Could you check a few things on this drawing? It's one solid part, dimensions in mm from its lowest x, y, z. Give positions to 0.01 mm unless a question says otherwise; leave off trailing zeros. Use a Markdown table: item, result.
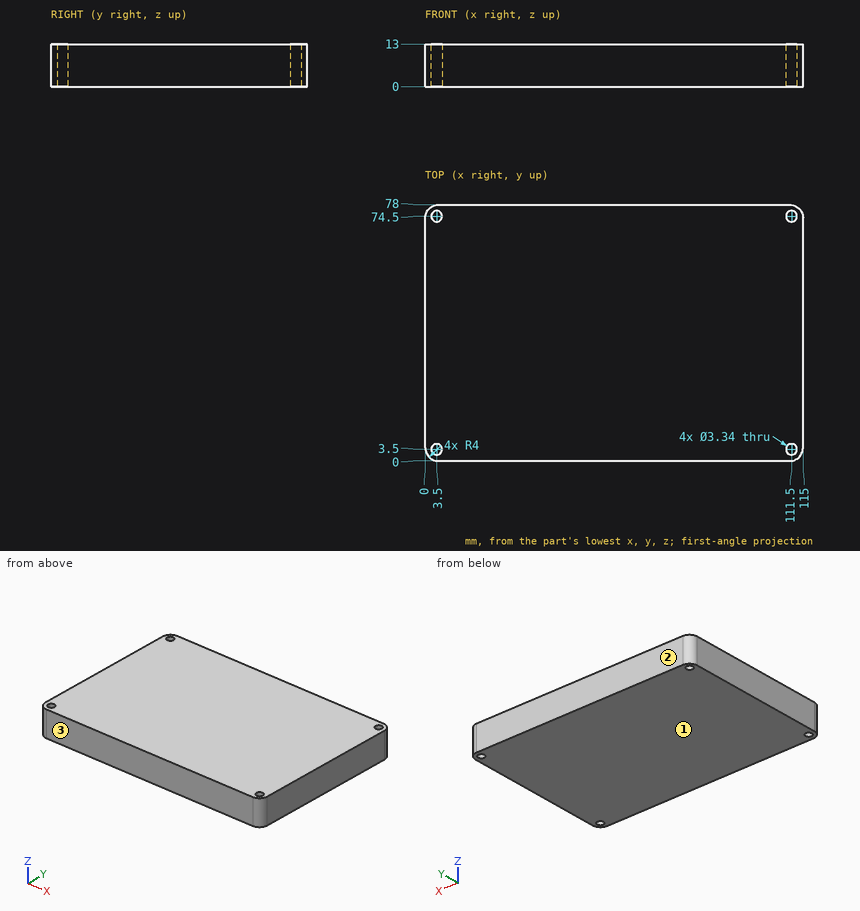
(1) We'd pull the mould along Y, two halves only. Please class the marked faces 1, 2 and 3: pulls with the +Y half, pulls with the -Y half, needs draft (parallel to the pull), parting line crosses it, or undercut.
A:
| item | result |
|---|---|
| face 1 | needs draft |
| face 2 | pulls with the +Y half |
| face 3 | pulls with the -Y half |
(2) Will this pin go through, and if not, where does the flat tip stop? pin 1 (2.5 mm diameter, centred on x = 3.5, y = 74.5, fed in from +Z).
A:
| item | result |
|---|---|
| pin 1 | through |
(3) If I drill on line 1 (X direction, y = 74.5, z = 6); line 2 (Y direction, x = 111.5, z = 7.5); line 3 (X direction, y = 75.5, z = 7.75), over which ranges is the centre line in solid material (lowest first)?
A:
| item | result |
|---|---|
| line 1 | 0.03 to 1.83, 5.17 to 109.83, 113.17 to 114.97 |
| line 2 | 0.03 to 1.83, 5.17 to 72.83, 76.17 to 77.97 |
| line 3 | 0.29 to 2.16, 4.84 to 110.16, 112.84 to 114.71 |
